from build123d import *

# Parameters (mm, degrees)
SKETCH1_W           = 63.5
SKETCH1_H           = 114.3
SKETCH1_W_2         = 38.1
SKETCH1_H_2         = 69.85
SKETCH1_W_3         = 50.8
SKETCH1_H_3         = 27.94
BOSS_EXTRUDE1_DEPTH = 19.05
SKETCH1_4_W         = 50.8
SKETCH1_4_H         = 27.94
CUT_EXTRUDE1_DEPTH  = 17.78
SKETCH3_W           = 8.203339587
SKETCH3_H           = 4.126489459
CUT_EXTRUDE2_DEPTH  = 17.78
SKETCH1_6_W         = 38.1
SKETCH1_6_H         = 69.85
CUT_EXTRUDE4_DEPTH  = 17.78
SKETCH7_W           = 5.588
SKETCH7_H           = 4.749156964
SKETCH7_W_2         = 6.35
SKETCH7_H_2         = 6.35
BOSS_EXTRUDE2_DEPTH = 11.43
CUT_EXTRUDE5_START  = 11.43
SKETCH6_R           = 1.598803
CUT_EXTRUDE5_DEPTH  = 7.62
FILLET2_R           = 6.35
CUT_EXTRUDE6_START  = -2.54
CUT_EXTRUDE6_DEPTH  = 2.54


with BuildPart() as part:
    # Sketch1 → Boss-Extrude1 (new body)
    # profile 1 of 3: a face of its own
    with BuildSketch(Plane.XY):
        with Locations((31.75, -57.15)):
            Rectangle(SKETCH1_W, SKETCH1_H)
        with Locations((31.75, -39.50921232)):
            Rectangle(SKETCH1_W_2, SKETCH1_H_2, mode=Mode.SUBTRACT)
        with Locations((31.75, -92.530701779)):
            Rectangle(SKETCH1_W_3, SKETCH1_H_3, mode=Mode.SUBTRACT)
    # profile 2 of 3: a face of its own
    with BuildSketch(Plane.XY):
        with Locations((31.75, -39.50921232)):
            Rectangle(SKETCH1_W_2, SKETCH1_H_2)
    # profile 3 of 3: a face of its own
    with BuildSketch(Plane.XY):
        with Locations((31.75, -92.530701779)):
            Rectangle(SKETCH1_W_3, SKETCH1_H_3)
    extrude(amount=BOSS_EXTRUDE1_DEPTH)

    # Sketch1<4> → Cut-Extrude1 (cut)
    with BuildSketch(Plane.XY):
        with Locations((31.75, -92.530701779)):
            Rectangle(SKETCH1_4_W, SKETCH1_4_H)
    extrude(amount=CUT_EXTRUDE1_DEPTH, mode=Mode.SUBTRACT)

    # Sketch3 → Cut-Extrude2 (cut)
    with BuildSketch(Plane(origin=(0, 0, 0), x_dir=(-1, 0, 0), z_dir=(0, 0, -1))):
        with Locations((-46.698330207, -76.497457049)):
            Rectangle(SKETCH3_W, SKETCH3_H)
    extrude(amount=-CUT_EXTRUDE2_DEPTH, mode=Mode.SUBTRACT)

    # Sketch1<6> → Cut-Extrude4 (cut)
    with BuildSketch(Plane.XY):
        with Locations((31.75, -39.50921232)):
            Rectangle(SKETCH1_6_W, SKETCH1_6_H)
    extrude(amount=CUT_EXTRUDE4_DEPTH, mode=Mode.SUBTRACT)

    # Sketch7 → Boss-Extrude2 (add)
    with BuildSketch(Plane(origin=(0, 0, 17.78), x_dir=(-1, 0, 0), z_dir=(0, 0, -1))):
        with Locations((-48.006, -70.764233838)):
            Rectangle(SKETCH7_W, SKETCH7_H)
        with Locations((-15.875, -71.25921232)):
            Rectangle(SKETCH7_W_2, SKETCH7_H_2)
        with Locations((-15.875, -7.75921232)):
            Rectangle(SKETCH7_W_2, SKETCH7_H_2)
        with Locations((-47.625, -7.75921232)):
            Rectangle(SKETCH7_W_2, SKETCH7_H_2)
    extrude(amount=BOSS_EXTRUDE2_DEPTH)

    # Sketch6 → Cut-Extrude5 (cut)
    with BuildSketch(Plane(origin=(0, 0, 17.78), x_dir=(-1, 0, 0), z_dir=(0, 0, -1)).offset(CUT_EXTRUDE5_START)):
        with Locations((-47.879, -70.59881232)):
            Circle(SKETCH6_R)
        with Locations((-16.0782, -70.59881232)):
            Circle(SKETCH6_R)
        with Locations((-47.879, -8.39421232)):
            Circle(SKETCH6_R)
        with Locations((-16.0782, -8.39421232)):
            Circle(SKETCH6_R)
    extrude(amount=-CUT_EXTRUDE5_DEPTH, mode=Mode.SUBTRACT)

    # Fillet2
    fillet2_edges = [part.edges().sort_by_distance(p)[0] for p in [
        (63.5, -114.3, 9.525),
        (0, -114.3, 9.525),
        (0, 0, 9.525),
        (63.5, 0, 9.525),
    ]]
    fillet(fillet2_edges, radius=FILLET2_R)

    # Sketch9 → Cut-Extrude6 (cut)
    with BuildSketch(Plane(origin=(0, 0, 0), x_dir=(-1, 0, 0), z_dir=(0, 0, -1)).offset(CUT_EXTRUDE6_START)):
        with BuildLine():
            ThreePointArc((-6.35, -114.3), (-1.859871939, -112.440128061), (0, -107.95))
            Line((0, -107.95), (0, -6.35))
            ThreePointArc((0, -6.35), (-1.859871939, -1.859871939), (-6.35, 0))
            Line((-6.35, 0), (-57.15, 0))
            ThreePointArc((-57.15, 0), (-61.640128061, -1.859871939), (-63.5, -6.35))
            Line((-63.5, -6.35), (-63.5, -107.95))
            ThreePointArc((-63.5, -107.95), (-61.640128061, -112.440128061), (-57.15, -114.3))
            Line((-57.15, -114.3), (-6.35, -114.3))
        make_face()
        with BuildLine():
            ThreePointArc((-60.96, -107.95), (-59.844076836, -110.644076836), (-57.15, -111.76))
            Line((-57.15, -111.76), (-6.35, -111.76))
            ThreePointArc((-6.35, -111.76), (-3.655923164, -110.644076836), (-2.54, -107.95))
            Line((-2.54, -107.95), (-2.54, -6.35))
            ThreePointArc((-2.54, -6.35), (-3.655923164, -3.655923164), (-6.35, -2.54))
            Line((-6.35, -2.54), (-57.15, -2.54))
            ThreePointArc((-57.15, -2.54), (-59.844076836, -3.655923164), (-60.96, -6.35))
            Line((-60.96, -6.35), (-60.96, -107.95))
        make_face(mode=Mode.SUBTRACT)
    extrude(amount=CUT_EXTRUDE6_DEPTH, mode=Mode.SUBTRACT)


solid = part.part
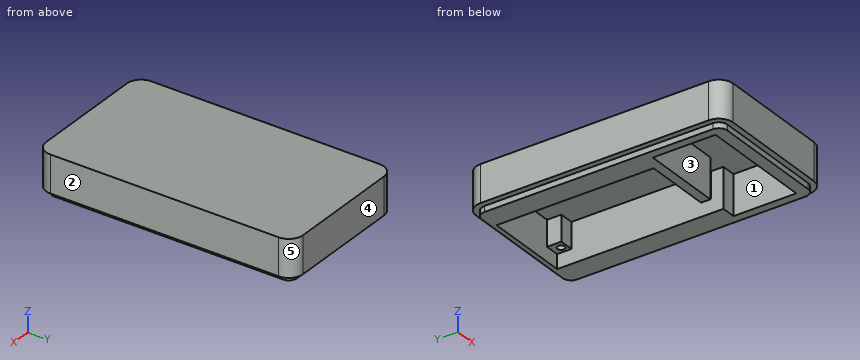
Design review of the part built by this model. Coordinates are the model's own, in mm. Face numbers are marked on the shaded views. A direction names the side the tool comes from. Round coordinates to 2 decimals unless told otherwise and drop trailing zeros. Loops run counter-clockwise (first coordinate to the right, second up) from the corner with the lowest first, then second, coordinate; pieces in that order, holes last. Notation, with made-up numbers: (-10.5, -36) - (12.5, -36) arc R18 ccw to (12.5, -20) - close; hole circle Ø8 at (57, 74.25). An arc over 180 degrees is marked (long way). One line per item, written item: value. Start each with the question number.
1) Consider section B-B on y = -77.5. Give the boundary of the cut face in (x, z).
2) Consider section D-D on z = 16.5. Give the boundary of the cut face in (x, y).
3) Consider section A-A on z = 4.5. Give the boundary of the cut face in (x, y).
4) Insertion check: pin 1 Ø2.5 at (x, y) = (49.5, -70) entering from -Z; pin 2 Ø5 at (x, y) = (34, -93) entering from -Z; pin 3 Ø0.8 at (y, z) = (-73, 1) entering from +X. Each pin has a flat end and moves straight along its axis. Give the tip position at first contact, or say it passes through.
5) Consider section C-C on x = 23.5. Give the boundary of the cut face in (y, z), then the cut area to 3 significant figures.
6) Draft analysis for pull direction X (two halves, no side actions). For the marked faces 3, 4 and 5, state which applies: +X half, -X half, draft (parallel to the pull), parting line (faces both ways), or undercut.
7) For the marked faces 1 and 2, list the 3-axis set-ups (+Z, -Z, +X, -X, +Y, -Y) from which the entire face can be reached by the end or side of a thin tool; tool diameter is ignored.
8) To check wall thickness, follow L1, parallel to Y at x = 24.5, z = 16; L2, parallel to Y at x = 45.5, z = 7.75; L3, parallel to X at y = -29.5, z = 12.75. State the ranges of each line that lie inside material, in increasing order. Write a range as from..to.
Reported:
1. outline: (0, 2.54) - (2.54, 2.54) - (2.54, 0) - (42.6, 0) - (42.6, 17.78) - (50.8, 17.78) - (50.8, 0) - (60.96, 0) - (60.96, 2.54) - (63.5, 2.54) - (63.5, 19.05) - (0, 19.05) - close
2. outline: (0, -107.95) arc R6.35 ccw to (6.35, -114.3) - (57.15, -114.3) arc R6.35 ccw to (63.5, -107.95) - (63.5, -6.35) arc R6.35 ccw to (57.15, 0) - (6.35, 0) arc R6.35 ccw to (0, -6.35) - close; hole (6.35, -106.5) - (57.15, -106.5) - (57.15, -78.56) - (50.8, -78.56) - (50.8, -73.14) - (45.21, -73.14) - (45.21, -68.39) - (50.8, -68.39) - (50.8, -10.93) - (44.45, -10.93) - (44.45, -4.58) - (19.05, -4.58) - (19.05, -10.93) - (12.7, -10.93) - (12.7, -68.08) - (19.05, -68.08) - (19.05, -74.43) - (42.6, -74.43) - (42.6, -78.56) - (6.35, -78.56) - close
3. outline: (0, -107.95) arc R6.35 ccw to (6.35, -114.3) - (57.15, -114.3) arc R6.35 ccw to (63.5, -107.95) - (63.5, -6.35) arc R6.35 ccw to (57.15, 0) - (6.35, 0) arc R6.35 ccw to (0, -6.35) - close; hole (6.35, -106.5) - (57.15, -106.5) - (57.15, -78.56) - (50.8, -78.56) - (50.8, -4.58) - (12.7, -4.58) - (12.7, -74.43) - (42.6, -74.43) - (42.6, -78.56) - (6.35, -78.56) - close
4. pin 1: stops at z = 6.35
4. pin 2: stops at z = 17.78
4. pin 3: stops at x = 60.96
5. outline: (-114.3, 2.54) - (-111.76, 2.54) - (-111.76, 0) - (-106.5, 0) - (-106.5, 17.78) - (-78.56, 17.78) - (-78.56, 0) - (-74.43, 0) - (-74.43, 17.78) - (-4.58, 17.78) - (-4.58, 0) - (-2.54, 0) - (-2.54, 2.54) - (0, 2.54) - (0, 19.05) - (-114.3, 19.05) - close
5. area: 426 mm^2
6. face 3: undercut
6. face 4: draft
6. face 5: +X half
7. face 1: -Z
7. face 2: +Z, -Z, +X, +Y, -Y
8. L1: y = -114.3..-106.5, -78.56..-74.43, -4.58..0
8. L2: y = -114.3..-106.5, -73.14..-68.39, -10.93..0
8. L3: x = 0..12.7, 50.8..63.5
